from build123d import *

# Parameters (mm, degrees)
SKETCH1_R                       = 60.96
BILLET_DEPTH                    = 12.7
SKETCH4_R                       = 0.7493
FIRST_KEROSENE_OUTLET_DEPTH     = 88.140881336
PRIMARY_HOLES_COUNT             = 6
SECOND_START                    = -12.7
SECOND_RING_OUTLINE_R           = 0.7493
SECOND_RING_DEPTH               = 12.7
THIRD_START                     = -12.7
THIRD_RING_OUTLINE_R            = 0.7493
THIRD_RING_DEPTH                = 12.7
SKETCH18_RX                     = 46.67504
SKETCH18_RY                     = 22.225
KEROSENE_WELL_DEPTH             = 9.3218
SKETCH17_R                      = 6.35
BOSS_EXTRUDE1_DEPTH             = 2.54
BOSS_EXTRUDE1_DIRECTION_2_REACH = 89.141
SKETCH21_R                      = 6.35
CUT_EXTRUDE1_DEPTH              = 2.54


# Read off the part's stored shape, not the designer's step: Second ring, Third Ring
with BuildPart() as part:
    # Sketch1 → Billet (new body)
    with BuildSketch(Plane(origin=(0, 0, 0), x_dir=(1, 0, 0), z_dir=(0, 1, 0))):
        with Locations(Location((0, 0, 0), (0, 0, 270))):
            Circle(SKETCH1_R)
    extrude(amount=-BILLET_DEPTH)

    # Sketch4 → First Kerosene Outlet (cut, symmetric)
    with BuildSketch(Plane(origin=(0, -12.7, 0), x_dir=(1, 0, 0), z_dir=(0, 1, 0))):
        with Locations(Location((8.9916, 0, 0), (0, 0, 270))):
            Circle(SKETCH4_R)
        with Locations(Location((13.4874, 0, 0), (0, 0, 270))):
            Circle(SKETCH4_R)
        with Locations(Location((17.9832, 0, 0), (0, 0, 270))):
            Circle(SKETCH4_R)
    first_kerosene_outlet = extrude(amount=FIRST_KEROSENE_OUTLET_DEPTH, both=True, mode=Mode.SUBTRACT)

    # Primary Holes: First Kerosene Outlet ×6 about axis
    primary_holes_axis = Axis((0, 0, 0), (0, 1, 0))
    for i in range(1, PRIMARY_HOLES_COUNT):
        add(first_kerosene_outlet.rotate(primary_holes_axis, i * 360 / PRIMARY_HOLES_COUNT), mode=Mode.SUBTRACT)

    # Second ring outline → Second ring (cut)
    with BuildSketch(Plane(origin=(0, 0, 0), x_dir=(1, 0, 0), z_dir=(0, 1, 0)).offset(SECOND_START)):
        with Locations((11.680431031, 6.7437)):
            Circle(SECOND_RING_OUTLINE_R)
        with Locations((0, 13.4874)):
            Circle(SECOND_RING_OUTLINE_R)
        with Locations((-11.680431031, 6.7437)):
            Circle(SECOND_RING_OUTLINE_R)
        with Locations((-11.680431031, -6.7437)):
            Circle(SECOND_RING_OUTLINE_R)
        with Locations((0, -13.4874)):
            Circle(SECOND_RING_OUTLINE_R)
        with Locations((11.680431031, -6.7437)):
            Circle(SECOND_RING_OUTLINE_R)
    extrude(amount=SECOND_RING_DEPTH, mode=Mode.SUBTRACT)

    # Third Ring outline → Third Ring (cut)
    with BuildSketch(Plane(origin=(0, 0, 0), x_dir=(1, 0, 0), z_dir=(0, 1, 0)).offset(THIRD_START)):
        with Locations((17.370437319, 4.654394652)):
            Circle(THIRD_RING_OUTLINE_R)
        with Locations((15.573908041, 8.9916)):
            Circle(THIRD_RING_OUTLINE_R)
        with Locations((12.716042667, 12.716042667)):
            Circle(THIRD_RING_OUTLINE_R)
        with Locations((4.654394652, 17.370437319)):
            Circle(THIRD_RING_OUTLINE_R)
        with Locations((0, 17.9832)):
            Circle(THIRD_RING_OUTLINE_R)
        with Locations((-4.654394652, 17.370437319)):
            Circle(THIRD_RING_OUTLINE_R)
        with Locations((-12.716042667, 12.716042667)):
            Circle(THIRD_RING_OUTLINE_R)
        with Locations((-15.573908041, 8.9916)):
            Circle(THIRD_RING_OUTLINE_R)
        with Locations((-17.370437319, 4.654394652)):
            Circle(THIRD_RING_OUTLINE_R)
        with Locations((-17.370437319, -4.654394652)):
            Circle(THIRD_RING_OUTLINE_R)
        with Locations((-15.573908041, -8.9916)):
            Circle(THIRD_RING_OUTLINE_R)
        with Locations((-12.716042667, -12.716042667)):
            Circle(THIRD_RING_OUTLINE_R)
        with Locations((-4.654394652, -17.370437319)):
            Circle(THIRD_RING_OUTLINE_R)
        with Locations((0, -17.9832)):
            Circle(THIRD_RING_OUTLINE_R)
        with Locations((4.654394652, -17.370437319)):
            Circle(THIRD_RING_OUTLINE_R)
        with Locations((12.716042667, -12.716042667)):
            Circle(THIRD_RING_OUTLINE_R)
        with Locations((15.573908041, -8.9916)):
            Circle(THIRD_RING_OUTLINE_R)
        with Locations((17.370437319, -4.654394652)):
            Circle(THIRD_RING_OUTLINE_R)
    extrude(amount=THIRD_RING_DEPTH, mode=Mode.SUBTRACT)

    # Sketch18 → Kerosene Well (cut)
    with BuildSketch(Plane(origin=(0, 0, 0), x_dir=(1, 0, 0), z_dir=(0, 1, 0))):
        with Locations(Location((0, 0), (0, 0, -180))):
            Ellipse(SKETCH18_RX, SKETCH18_RY)
    extrude(amount=-KEROSENE_WELL_DEPTH, mode=Mode.SUBTRACT)

    # Sketch17 → Boss-Extrude1 (add)
    with BuildSketch(Plane(origin=(0, 0, 0), x_dir=(1, 0, 0), z_dir=(0, 1, 0))):
        with Locations(Location((0, 0, 0), (0, 0, 270))):
            Circle(SKETCH17_R)
    extrude(amount=BOSS_EXTRUDE1_DEPTH)

    # Sketch17 → Boss-Extrude1 direction 2 (add, up to next)
    with BuildSketch(Plane(origin=(0, 0, 0), x_dir=(1, 0, 0), z_dir=(0, 1, 0)), mode=Mode.PRIVATE) as boss_extrude1_direction_2_sk1:
        with Locations(Location((0, 0, 0), (0, 0, 270))):
            Circle(SKETCH17_R)
    boss_extrude1_direction_2_tool1 = extrude(boss_extrude1_direction_2_sk1.sketch, amount=-BOSS_EXTRUDE1_DIRECTION_2_REACH, mode=Mode.PRIVATE) - part.part
    add(boss_extrude1_direction_2_tool1.solids().sort_by_distance((0, 0, 0))[0])

    # Sketch21 → Cut-Extrude1 (cut)
    with BuildSketch(Plane(origin=(0, 2.54, 0), x_dir=(1, 0, 0), z_dir=(0, 1, 0))):
        with Locations(Location((0, 0, 0), (0, 0, 270))):
            Circle(SKETCH21_R)
    extrude(amount=-CUT_EXTRUDE1_DEPTH, mode=Mode.SUBTRACT)


solid = part.part
Part model, mm, in its own coordinate system. A direction names the side the tool comes from. Coordinates: 2 decimals unless noted, no trailing zeros. Order: outer loops, then holes, each group sorted by start corner. A loop starts at its lowest first (then second) coordinate and runs counter-clockwise, first axis right, second up.
(1) Tool access for faces 4 (the face through (-10, -9.322, 0)), 5 (the face through (1, -12.7, -1)): list every direction of +Z, -Z, +X, -X, +Y, -Y with a clear straight run to the whole face (end or side of a thin tool).
Check sheet entries:
face 4: +Y
face 5: +Z, -Z, +X, -X, -Y
(2) Slice it at A-A, the plane y = -10.75. State how many separate pieces and enclosed holes the cut face has, and give its area (3 significant figures).
Check sheet entries:
separate pieces: 1
enclosed holes: 42
area: 11,600 mm2
(3) Slice it at B-B, the plane z = -50. Write the cut outline in (x, y), and give its area (3 significant figures).
Check sheet entries:
outline: (-34.87, -12.7) - (34.87, -12.7) - (34.87, 0) - (-34.87, 0) - close
area: 886 mm2
(4) Pull direction Z, two halves, no side cores. Call faces 1 (the face through (0, 0, 0)), 2 (the face through (60.44, -6.26, -7.94)), 3 (the face through (-3.86, -4.6, -5.04)): pulls with the +Z half, pulls with the -Z half, needs draft (parallel to the pull), parting line crosses it, or undercut.
Check sheet entries:
face 1: needs draft
face 2: parting line crosses it
face 3: undercut
(5) Probe L1, parallel to Z at x = -7, y = -3.5; L2, parallel to Y at x = -41, z = 7; L3, parallel to Z at x = -31, y = -8.75. List the from-to ranges inside material, lowest first.
Check sheet entries:
L1: z = -60.56 to -21.97, 21.97 to 60.56
L2: y = -12.7 to -9.32
L3: z = -52.49 to -16.62, 16.62 to 52.49
(6) Pin check, flat tips, straight feed: pin 1 Ø3 at (y, z) = (-8.5, -28) entering from -X; pin 2 Ø1.5 at (x, y) = (39, -7) entering from +Z; pin 3 Ø1.5 at (x, y) = (45, -4.5) entering from -Z. Stop position of each tip, or through.
Check sheet entries:
pin 1: stops at x = -54.9
pin 2: stops at z = 47.47
pin 3: stops at z = -41.93
